Source: CAD feature listing. Evaluate the final solid. Frame: model axes, mm. Face numbers are marked on the shaded views. A direction names the side the tool comes from. Round coordinates to 2 decimals unless told otherwise and drop trailing zeros. Loops run counter-clockwise (first coordinate to the right, second up) from the corner with the lowest first, then second, coordinate; pieces in that order, holes last.
Item 1: Section query A-A on z = 4.4. Return loops of the section in (x, y) (3 decimals), then the cut area to 3 significant figures.
Item 2: First-contact query: P1, Ø3, axis at x = 20.5, y = 30.9, coming from the -Z side; P2, Ø2, axis at y = 8, z = 2.5, coming from the +X side; P3, Ø1.5, axis at y = 26, z = 1, coming from the +X side. Flat tips, straight axial feed; report the tip coordinate or a pass-through.
Item 3: Access query for the marked faces 1 and 2. Directions: +Z, -Z, +X, -X, +Y, -Y. A direction counts if a zero-diameter tool reaches every point of the face in a straight line with its end or side. Return the directions, or none.
Item 4: Section query C-C on x = 12. Return loops of the section in (y, z), then the cut area to 3 significant figures.
Item 5: Ray query, L1, parallel to Y at x = 20.5, z = 3.5; L2, parallel to X at y = 31, z = 0.2; L3, parallel to Y at x = 12, z = 3.5. Return the intervals inside material, ascending.
Item 6: Section query B-B on y = 17. Return loops of the section in (x, z), then the cut area to 3 significant figures.
Item 7: Section query D-D on y = 21.4. Return loops of the section in (x, z).
```python
from build123d import *

# Parameters (mm, degrees)
BOSS_EXTRUDE1_DEPTH       = 4.826
M3X0_5_TAPPED_HOLE2_D     = 2.5
M3X0_5_TAPPED_HOLE3_D     = 2.5
M3X0_5_TAPPED_HOLE3_DEPTH = 5
M3X0_5_TAPPED_HOLE3_TIP   = 0.751075774
FILLET2_R                 = 4
M3X0_5_TAPPED_HOLE4_D     = 2.5
M3X0_5_TAPPED_HOLE5_D     = 2.5


with BuildPart() as part:
    # Sketch1 → Boss-Extrude1 (new body)
    with BuildSketch(Plane.XY):
        Polygon((0, 0), (0, 13.5), (8, 36.5), (23, 36.5), (23, 8.5), (35, 8.5), (35, 0), align=None)
    extrude(amount=BOSS_EXTRUDE1_DEPTH)

    # M3x0.5 Tapped Hole2 (through all)
    with Locations(Plane.XY.offset(4.826)):
        with Locations((12, 31.9)):
            Hole(M3X0_5_TAPPED_HOLE2_D / 2)

    # M3x0.5 Tapped Hole3
    with Locations(Plane(origin=(0, 0, 0), x_dir=(-1, 0, 0), z_dir=(0, -1, 0))):
        with Locations((-16.73, -2.413), (-28.73, -2.413)):
            Hole(M3X0_5_TAPPED_HOLE3_D / 2, depth=M3X0_5_TAPPED_HOLE3_DEPTH)
            with Locations((0, 0, -(M3X0_5_TAPPED_HOLE3_DEPTH + M3X0_5_TAPPED_HOLE3_TIP / 2))):  # 118° drill point
                Cone(0, M3X0_5_TAPPED_HOLE3_D / 2, M3X0_5_TAPPED_HOLE3_TIP, mode=Mode.SUBTRACT)

    # Fillet2
    fillet2_edges = [part.edges().sort_by_distance(p)[0] for p in [
        (23, 36.5, 2.413),
        (23, 8.5, 2.413),
        (35, 8.5, 2.413),
        (0, 13.5, 2.413),
        (8, 36.5, 2.413),
    ]]
    fillet(fillet2_edges, radius=FILLET2_R)

    # M3x0.5 Tapped Hole4 (through all)
    with Locations(Plane.XY.offset(4.826)):
        with Locations((19.5, 21.4), (20.5, 30.9)):
            Hole(M3X0_5_TAPPED_HOLE4_D / 2)

    # M3x0.5 Tapped Hole5 (through all)
    with Locations(Plane.XY.offset(4.826)):
        with Locations((11.425, 16.46), (11.425, 10.46)):
            Hole(M3X0_5_TAPPED_HOLE5_D / 2)


solid = part.part
```
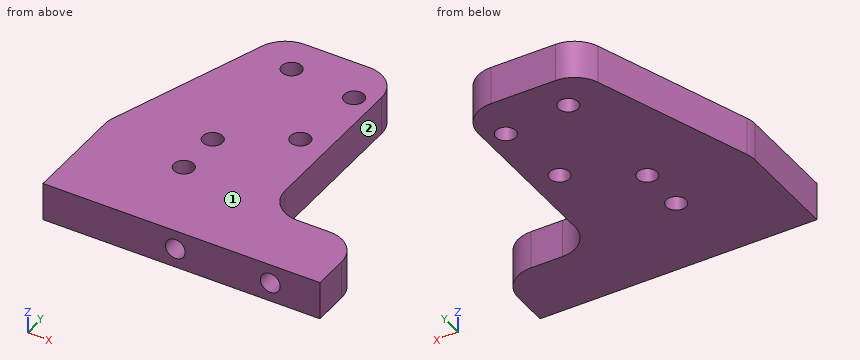
Data:
1. outline: (0, 0) - (35, 0) - (35, 4.5) arc R4 ccw to (31, 8.5) - (27, 8.5) arc R4 cw to (23, 12.5) - (23, 32.5) arc R4 ccw to (19, 36.5) - (10.844, 36.5) arc R4 ccw to (7.066, 33.814) - (0.222, 14.138) arc R4 ccw to (0, 12.824) - close; hole circle Ø2.5 at (11.425, 10.46); hole circle Ø2.5 at (11.425, 16.46); hole circle Ø2.5 at (12, 31.9); hole circle Ø2.5 at (19.5, 21.4); hole circle Ø2.5 at (20.5, 30.9)
1. area: 820 mm2
2. P1: stops at z = 0
2. P2: stops at x = 34.12
2. P3: stops at x = 23
3. face 1: +Z, +X, -X, +Y, -Y
3. face 2: +Z, -Z, +X, +Y
4. outline: (0, 0) - (9.35, 0) - (9.35, 4.83) - (0, 4.83) - close; (11.57, 0) - (15.35, 0) - (15.35, 4.83) - (11.57, 4.83) - close; (17.57, 0) - (30.65, 0) - (30.65, 4.83) - (17.57, 4.83) - close; (33.15, 0) - (36.5, 0) - (36.5, 4.83) - (33.15, 4.83) - close
4. area: 143 mm2
5. L1: y = 0 to 20.65, 22.15 to 29.65, 32.15 to 36.21
5. L2: x = 6.09 to 11.13, 12.87 to 19.25, 21.75 to 23
5. L3: y = 0 to 9.35, 11.57 to 15.35, 17.57 to 30.65, 33.15 to 36.5
6. outline: (1.22, 0) - (10.3, 0) - (10.3, 4.83) - (1.22, 4.83) - close; (12.55, 0) - (23, 0) - (23, 4.83) - (12.55, 4.83) - close
6. area: 94.2 mm2
7. outline: (2.75, 0) - (18.25, 0) - (18.25, 4.83) - (2.75, 4.83) - close; (20.75, 0) - (23, 0) - (23, 4.83) - (20.75, 4.83) - close
